Verification items for this drawing (mm, ordinates from the low corner). Give positions to 0.01 mm unless a question says otherwise; leave off trailing zeros. Loops run counter-clockwise (first coordinate to the right, second up) from the corner with the lowest first, then second, coordinate; pieces in that order, holes last. Notation, with made-up numbers: M 5.25,-13.75 L 31.25,-13.75 A20 ccw 31.25,12.25 Z; hole C 30.25,56 d8. An arc over 180 degrees is marked long. Answer in a Markdown table with one row per item.
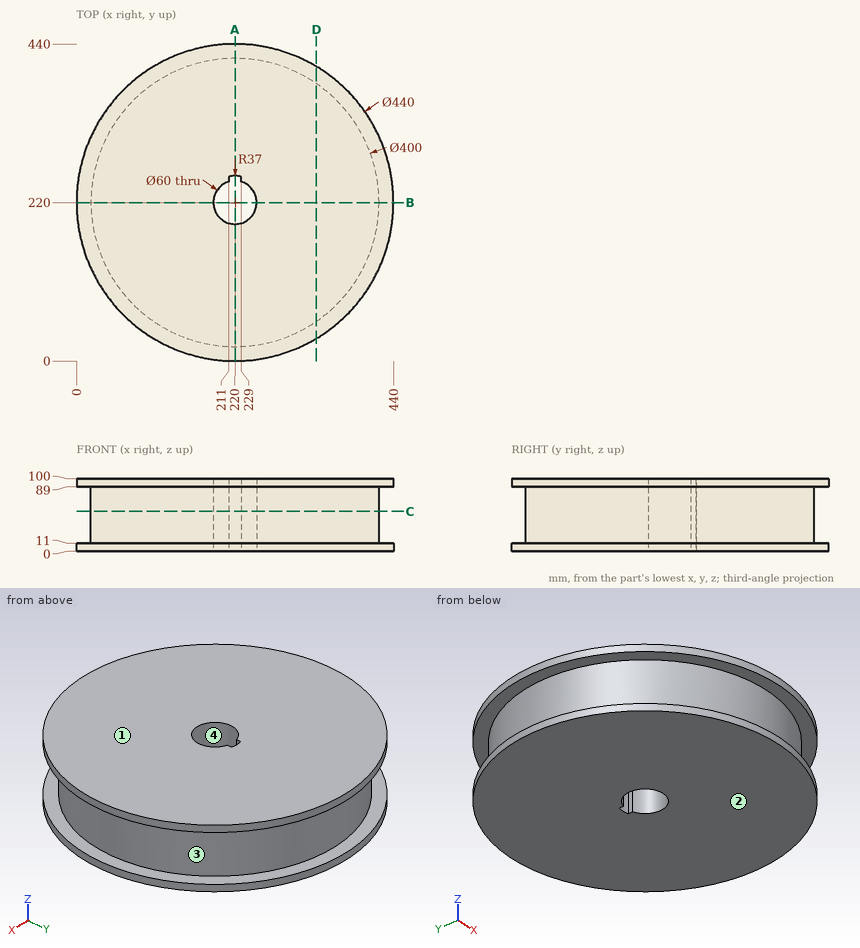
Item 1: Sectioned sample at C-C (z = 55). Record the cut outline in (x, y), and give its area (3 significant figures).
Reported:
| item | result |
|---|---|
| outline | C 220,220 d400; hole M 211,248.62 A30 ccw long 229,248.62 L 229,255.89 A37 ccw 211,255.89 Z |
| area | 123,000 mm^2 |
Item 2: Sectioned sample at B-B (y = 220). Record the cut outline in (x, z).
Reported:
| item | result |
|---|---|
| outline | M 0,0 L 190,0 L 190,100 L 0,100 L 0,89 L 20,89 L 20,11 L 0,11 Z; M 250,0 L 440,0 L 440,11 L 420,11 L 420,89 L 440,89 L 440,100 L 250,100 Z |
Item 3: Sectioned sample at D-D (x = 333). Record the cut outline in (y, z), and give its area (3 significant figures).
Reported:
| item | result |
|---|---|
| outline | M 31.24,0 L 408.76,0 L 408.76,11 L 385.02,11 L 385.02,89 L 408.76,89 L 408.76,100 L 31.24,100 L 31.24,89 L 54.98,89 L 54.98,11 L 31.24,11 Z |
| area | 34,000 mm^2 |
Item 4: Sectioned sample at A-A (x = 220). Record the cut outline in (y, z).
Reported:
| item | result |
|---|---|
| outline | M 0,0 L 190,0 L 190,100 L 0,100 L 0,89 L 20,89 L 20,11 L 0,11 Z; M 257,0 L 440,0 L 440,11 L 420,11 L 420,89 L 440,89 L 440,100 L 257,100 Z |
Item 5: Release check for a two-part mould opening along Z. For the marked faces 1, 2, 3 and 4 record: released by +Z, released by -Z, zero draft, split by the parting line, or undercut.
Reported:
| item | result |
|---|---|
| face 1 | released by +Z |
| face 2 | released by -Z |
| face 3 | undercut |
| face 4 | zero draft |
Item 6: Go/stop test with flat-tipped pins: pin 1 (8 mm diameter, centred on y = 252.5, z = 69.5, fed in from +X); pin 2 (8 mm diameter, centred on y = 190.5, z = 26.5, fed in from +X); pin 3 (4 mm diameter, centred on x = 95.5, z = 82.5, fed in from -Y). Record where each tip stops, or that it passes through.
Reported:
| item | result |
|---|---|
| pin 1 | stops at x = 417.96 |
| pin 2 | stops at x = 418.37 |
| pin 3 | stops at y = 61.91 |
Item 7: Scan lines: L1, parallel to Z at x = 391, y = 101.5; L2, parallel to Y at x = 220, z = 23.5; L3, parallel to Y at x = 198, z = 7. Record each from-to range of solid material in increasing order. Write a range as [from, to].
Reported:
| item | result |
|---|---|
| L1 | z = [0, 11], [89, 100] |
| L2 | y = [20, 190], [257, 420] |
| L3 | y = [1.1, 199.6], [240.4, 438.9] |
